```python
from build123d import *

# Parameters (mm, degrees)
F4_DEPTH  = 7.9385001
F5_W      = 3.1188364687
F5_H      = 16.0931088583
F6_DEPTH  = 7.9375
F7_R      = 1.8415
F8_DEPTH  = 3.1188364687
F9_R      = 1.8415
F10_DEPTH = 3.1188364687
F11_R     = 1.905


with BuildPart() as f2:
    # F1 (on Front) → F2 (revolve)
    with BuildSketch(Plane.XZ):
        with BuildLine():
            ThreePointArc((-13.0361579316, 7.9375), (-14.2875, 3.96875), (-13.0361579316, 0))
            Line((-13.0361579316, 0), (-11.1125, 0))
            Line((-11.1125, 0), (-11.1125, 7.9375))
            Line((-11.1125, 7.9375), (-13.0361579316, 7.9375))
        make_face()
    revolve(axis=Axis((0, 0, 3.96875), (0, 0, 1)))

    # F3 (on face) → F4 (cut, through all)
    with BuildSketch(Plane.XY.offset(7.9375)):
        with BuildLine():
            Line((-10.2775673973, -9.9249314679), (-9.3774272437, -9.0556762258))
            ThreePointArc((-9.3774272437, -9.0556762258), (-10.546473308, 7.6624613788), (5.7146755022, 11.7168211356))
            Line((5.7146755022, 11.7168211356), (6.2632277597, 12.8415199365))
            ThreePointArc((6.2632277597, 12.8415199365), (-11.5588303071, 8.3979817921), (-10.2775673973, -9.9249314679))
        make_face()
        with BuildLine():
            Line((-9.3774272437, -9.0556762258), (-7.9936635313, -7.7193911417))
            ThreePointArc((-7.9936635313, -7.7193911417), (-8.99020135, 6.5317636161), (4.8713993687, 9.9878488395))
            Line((4.8713993687, 9.9878488395), (5.7146755022, 11.7168211356))
            ThreePointArc((5.7146755022, 11.7168211356), (-10.546473308, 7.6624613788), (-9.3774272437, -9.0556762258))
        make_face()
    extrude(amount=-F4_DEPTH, mode=Mode.SUBTRACT)

    # F5 (on Top) → F6 (join, through all)
    with BuildSketch(Plane.XY):
        with Locations((-9.5530817656, -15.7659455709)):
            Rectangle(F5_W, F5_H)
        Polygon((20.1768554158, 14.960892969), (19.2130819443, 17.9270827159), (3.9076258972, 12.9540385864), (4.8713993687, 9.9878488395), align=None)
    extrude(amount=F6_DEPTH)

    # F7 (on face) → F8 (cut, through all)
    with BuildSketch(Plane.YZ.offset(-7.9936635313)):
        with BuildLine():
            ThreePointArc((-23.8125, 3.96875), (-23.4922534904, 6.0494249827), (-22.5611579316, 7.9375))
            Line((-22.5611579316, 7.9375), (-23.8125, 7.9375))
            Line((-23.8125, 7.9375), (-23.8125, 3.96875))
        make_face()
        with BuildLine():
            Line((-23.8125, 0), (-22.5611579316, 0))
            ThreePointArc((-22.5611579316, 0), (-23.4922534904, 1.8880750173), (-23.8125, 3.96875))
            Line((-23.8125, 3.96875), (-23.8125, 0))
        make_face()
        with Locations((-19.84375, 3.96875)):
            Circle(F7_R)
    extrude(amount=-F8_DEPTH, mode=Mode.SUBTRACT)

    # F9 (on face) → F10 (cut, through all)
    with BuildSketch(Plane(origin=(-2.4701778785, 7.6024257905, 0), x_dir=(0.9510565163, 0.3090169944, 0), z_dir=(0.3090169944, -0.9510565163, 0))):
        with Locations((19.84375, 3.96875)):
            Circle(F9_R)
        with BuildLine():
            ThreePointArc((22.5611579316, 7.9375), (23.4922534904, 6.0494249827), (23.8125, 3.96875))
            Line((23.8125, 3.96875), (23.8125, 7.9375))
            Line((23.8125, 7.9375), (22.5611579316, 7.9375))
        make_face()
        with BuildLine():
            ThreePointArc((23.8125, 3.96875), (23.4922534904, 1.8880750173), (22.5611579316, 0))
            Line((22.5611579316, 0), (23.8125, 0))
            Line((23.8125, 0), (23.8125, 3.96875))
        make_face()
    extrude(amount=-F10_DEPTH, mode=Mode.SUBTRACT)

    # F11
    f11_edges = [f2.edges().sort_by_distance(p)[0] for p in [
        (-7.993664, -11.842044, 3.96875),
        (8.792275, 11.261819, 3.96875),
    ]]
    fillet(f11_edges, radius=F11_R)


solid = f2.part
```
Source: CAD feature listing. Evaluate the final solid. Frame: model axes, mm. A direction names the side the tool comes from. Coordinates: 2 decimals unless noted, no trailing zeros. Order: outer loops, then holes, each group sorted by start corner. A loop starts at its lowest first (then second) coordinate and runs counter-clockwise, first axis right, second up. Notation, with made-up numbers: (46.25, -9.75) - (71.25, -9.75) arc R5 cw to (71.25, -3.75) - close; hole circle Ø4 at (72.25, -12). An arc over 180 degrees is marked (long way). One line per item, written item: value.
1) Reachability of faces 1 (the face through (-10, -7.719, 4)), 2 (the face through (4.383, 11.492, 3.913)), 3 (the face through (-9.531, -21.201, 5.213)) from +Z, -Z, +X, -X, +Y, -Y: full face, straight path, thin tool, end or side. Return the list, or none.
Computed values:
face 1: +Z, -Z, -X, +Y
face 2: +Z, -Z, -X
face 3: +X, -X
2) Ray query, line 1 (Y direction, x = 0, z = 6); line 2 (X direction, y = -16, z = 7); line 3 (X direction, y = -8.5, z = 7). Return the intervals inside material, ascending. Write a range as [from, to].
Computed values:
line 1: y = [-13.98, -11.11]
line 2: x = [-11.11, -7.99]
line 3: x = [-11.11, -7.16], [7.16, 10.6]
3) Cut plane A-A on z = 4.5. State how many separate pieces and enclosed holes the cut face has, plus the area to 3 significant figures.
Computed values:
separate pieces: 3
enclosed holes: 0
area: 213 mm^2
4) Cut plane B-B on x = 0. Output: boundary loops of the cut face in (y, z).
Computed values:
outline: (-13.04, 0) - (-11.11, 0) - (-11.11, 7.94) - (-13.04, 7.94) arc R6.92 ccw to start
5) Cut plane C-C on y = 0. Output: boundary loops of the cut face in (x, z), plus the area to 3 significant figures.
Computed values:
outline: (11.11, 0) - (13.04, 0) arc R6.92 ccw to (13.04, 7.94) - (11.11, 7.94) - close
area: 22.0 mm^2
6) Mould query, pull axis X, two halves, no side actions, for faces 4 (the face through (8.83, -6.75, 4.02)), 5 (the face through (14.396, 13.083, 3.913)), 6 (the face through (11, -4, 0)). Classes: released by +X, released by -X, zero draft, split by the parting line, or undercut.
Computed values:
face 4: undercut
face 5: released by +X
face 6: zero draft
7) Contact query for flat-ended pins moving along their axis: pin 1 (3 mm diameter, centred on x = 8, z = 5, fed in from -Y); pin 2 (3 mm diameter, centred on x = 6, z = 4, fed in from +Y); pin 3 (2.5 mm diameter, centred on x = -10, z = 3, fed in from +Y). Output: stop coordinate, or through.
Computed values:
pin 1: stops at y = -12.66
pin 2: stops at y = 14.12
pin 3: stops at y = -7.72
